Input: part model. Units: mm. Frame: model coordinates. A direction names the side the tool comes from. Coordinates: 2 decimals unless noted, no trailing zeros. Write each loop counter-clockwise with the first axis right and the second up, starting at its lowest first coordinate (ties: lowest second). Pieces come first, ordered by that corner, then holes. Notation, with made-up numbers: (62, -23) -> (71, -23) arc R15 ccw to (71, -8) -> close; hole circle Ø7 at (75.5, 34). An arc over 180 degrees is marked (long way). One line per question, with ' | ' between items. Start each with the question number.
Autodesk Inventor part; units mm, degrees
ref_plane "YZ Plane" through (0, 0, 0) normal (1, 0, 0) x (0, 1, 0)
ref_plane "XZ Plane" through (0, 0, 0) normal (0, 1, 0) x (-1, 0, 0)
ref_plane "XY Plane" through (0, 0, 0) normal (0, 0, 1) x (1, 0, 0)
sketch "Sketch1" plane through (0, 0, 0) normal (1, 0, 0) x (0, 1, 0)
  line L0 (0, 0) -> (50, 0)
  line L1 (50, 0) -> (50, 110)
  line L2 (50, 110) -> (0, 110)
  line L3 (0, 110) -> (0, 0)
  line L4 (50, 0) -> (0, -28.8675)
  line L5 (0, -28.8675) -> (0, 0)
  dimension "d0" = 110
  dimension "d1" = 50
  dimension "d68" = 60
extrude "Extrusion1" add sketch "Sketch1" along normal blind 5
fillet "Fillet1" radius 4 2 edges at (2.5, 50, 0) (2.5, 0, -28.8675)
sketch "Sketch2" plane through (5, 0, 0) normal (1, 0, 0) x (0, 0, -1)
  line L0 (-2.3094, 50) -> (-110, 50)
  line L1 (-110, 50) -> (-110, 0)
  line L2 (-110, 33.9915) -> (-75, 50)
  line L3 (-110, 16.0085) -> (-75, 0)
  line L4 (-110, 50) -> (-56.045, 50)
  line L5 (-56.045, 50) -> (-56.045, 0)
  line L6 (-56.045, 0) -> (-110, 0)
  line L7 (-110, 0) -> (-110, 50)
  line L8 (-110, 33.9915) -> (-110, 16.0085)
  line L9 (-110, 50) -> (-110, 0)
  line L10 (-110, 0) -> (-75, 0)
  circle A0 centre (-96, 25) radius 14
  circle A1 centre (-96, 25) radius 8.05
  line L11 (-96, 25) -> (-90.3078, 19.3078)
  line L12 (-96, 25) -> (-87.95, 25) construction
  circle A2 centre (-90.3078, 19.3078) radius 1.5
  circle A3 centre (-90.3078, 30.6922) radius 1.5
  circle A4 centre (-101.6922, 30.6922) radius 1.5
  circle A5 centre (-101.6922, 19.3078) radius 1.5
  point P0 (0, 0)
  point P1 (-110, 0)
  point P2 (-75, 0)
  point P3 (-110, 25)
  point P4 (-101.8232, 37.7315)
  point P5 (-101.8232, 12.2685)
  dimension "d84" = 16.1
  dimension "d13" = 35
  dimension "d82" = 28
  dimension "d83" = 25
  dimension "d86" = 45
  dimension "d87" = 3
  dimension "d90" = 360
extrude "Extrusion2" cut sketch "Sketch2" against normal blind 5 contours L2 L1 L0 | A0 L1 L2 | L6 L1 L3 | A0 L3 L1 | A3 A1 | A1 A3 | A2 A1 | A1 L11 A2 | A1 A2 L11 | A4 A1 | A1 A4 | A5 A1 | A1 A5
fillet "Fillet3" radius 4 1 edges at (2.5, 50, 75)
chamfer "Chamfer1" distance 2 angle 45 4 edges at (5, 30.6922, 91.8078) (5, 19.3078, 91.8078) (5, 19.3078, 103.1922) (5, 30.6922, 103.1922)
sketch "Sketch7" plane through (5, 0, 0) normal (1, 0, 0) x (0, 0, -1)
  circle A0 centre (-63, 43) radius 3
  circle A1 centre (-63, 7) radius 3
  circle A2 centre (14, 7) radius 3
  line L0 (-2.3094, 50) -> (-74.1286, 50)
  line L1 (-74.1286, 0) -> (21.9393, 0)
  point P0 (0, 0)
  dimension "d97" = 7
  dimension "d98" = 7
  dimension "d99" = 6
  dimension "d100" = 63
  dimension "d101" = 14
extrude "Extrusion7" cut sketch "Sketch7" against normal blind 10
sketch "Sketch8" plane through (5, 0, 0) normal (1, 0, 0) x (0, 0, -1)
  line L0 (-48.7321, 42) -> (-4.6188, 42)
  line L1 (-4.6188, 42) -> (-4.6188, 8)
  line L2 (-4.6188, 8) -> (-48.7321, 8)
  line L3 (-48.7321, 8) -> (-48.7321, 42)
  line L4 (-48.7321, 42) -> (-78.1769, 25)
  line L5 (-78.1769, 25) -> (-48.7321, 8)
  line L6 (-4.6188, 42) -> (5.1962, 25)
  line L7 (5.1962, 25) -> (-4.6188, 8)
  line L8 (25.4034, 6) -> (1.1547, 48)
  line L9 (-2.3094, 50) -> (-74.1286, 50)
  line L10 (-74.1286, 0) -> (21.9393, 0)
  circle A0 centre (-63, 43) radius 3
  point P0 (0, 0)
  dimension "d104" = 8
  dimension "d105" = 8
  dimension "d106" = 8
  dimension "d107" = 8
extrude "Extrusion8" cut sketch "Sketch8" against normal blind 10 contours L0 L1 L2 L3 | L3 L5 L4 | L6 L7 L1
fillet "Fillet5" radius 4 6 edges at (2.5, 25, 78.1769) (2.5, 42, 48.7321) (2.5, 42, 4.6188) (2.5, 25, -5.1962) (2.5, 8, 4.6188) (2.5, 8, 48.7321)
properties part number "frame_side"
1) Section C-C, the plane x = 1.75. Give the number of separate pieces and of enclosed holes in the cut face, then the cut area to 3 significant figures.
2) Section B-B, the plane z = 63. Return loops of the section in (x, y), then the cut area to 3 significant figures.
3) First-contact query: P1, Ø5, axis at y = 7, z = -14, coming from the +X side; P2, Ø3, axis at x = 2, z = 84, coming from the -Y side. Flat tips, straight axial feed; report the tip coordinate or a pass-through.
4) Section A-A, the plane z = 20.5. Return loops of the section in (x, y).
5) Ray query, line 1 (Y direction, x = 0.6, z = 8); line 2 (Y direction, x = 3, z = 63); line 3 (Z direction, x = 3.2, y = 31.5). Return the intervals inside material, ascending.
6) Section D-D, the plane z = -14. Return loops of the section in (x, y).
7) Access query for faces 1 (the face through (3.125, 19.796, 88.758)), 2 (the face through (3, 42, 28)). Directions: +Z, -Z, +X, -X, +Y, -Y. A direction counts if a zero-diameter tool reaches every point of the face in a straight line with its end or side. Return the directions, or none.
8) Pull-direction query (Z, two-part tool) for faces 3 (the face through (3, 25, 110)), 4 (the face through (5, 2, 43)), 5 (the face through (1.521, 19.758, 88.877)); classes: released by +Z, released by -Z, zero draft, split by the parting line, or undercut.
Answer block:
1) separate pieces: 1 | enclosed holes: 8 | area: 3,350 mm2
2) outline: (0, 0) -> (5, 0) -> (5, 4) -> (0, 4) -> close; (0, 10) -> (5, 10) -> (5, 16.24) -> (0, 16.24) -> close; (0, 33.76) -> (5, 33.76) -> (5, 40) -> (0, 40) -> close; (0, 46) -> (5, 46) -> (5, 50) -> (0, 50) -> close | area: 102 mm2
3) P1: passes through | P2: stops at y = 3.43
4) outline: (0, 0) -> (5, 0) -> (5, 8) -> (0, 8) -> close; (0, 42) -> (5, 42) -> (5, 50) -> (0, 50) -> close
5) line 1: y = 0 to 8, 42 to 50 | line 2: y = 0 to 4, 10 to 16.24, 33.76 to 40, 46 to 50 | line 3: z = -10.68 to -1.44, 66.92 to 88.81, 91.8 to 100.2, 103.19 to 108.4
6) outline: (0, 0) -> (5, 0) -> (5, 4) -> (0, 4) -> close; (0, 10) -> (5, 10) -> (5, 25.75) -> (0, 25.75) -> close
7) face 1: +X | face 2: +X, -X
8) face 3: released by +Z | face 4: zero draft | face 5: undercut
